from build123d import *

# Parameters (mm, degrees)
F0_R     = 8.382
F1_DEPTH = 12.7
F2_R     = 24.4449127013
F3_DEPTH = 25.4
F4_R     = 5.08
F6_DEPTH = 38.101


with BuildPart() as f1:
    # F0 (on Top) → F1 (new body)
    with BuildSketch(Plane.XY):
        with BuildLine():
            Line((10.7001249271, 26.4959987837), (0, 28.575))
            ThreePointArc((0, 28.575), (-28.575, 0), (0, -28.575))
            Line((0, -28.575), (10.7001249271, -26.4959987837))
            ThreePointArc((10.7001249271, -26.4959987837), (23.6884644373, -15.9808409542), (28.575, 0))
            ThreePointArc((28.575, 0), (23.6884644373, 15.9808409542), (10.7001249271, 26.4959987837))
        make_face()
        with BuildLine():
            ThreePointArc((10.7001249271, 26.4959987837), (5.4501128317, 28.0504348473), (0, 28.575))
            Line((0, 28.575), (10.7001249271, 26.4959987837))
        make_face()
        with BuildLine():
            Line((10.7001249271, -26.4959987837), (0, -28.575))
            ThreePointArc((0, -28.575), (5.4501128317, -28.0504348473), (10.7001249271, -26.4959987837))
        make_face()
        with BuildLine():
            Line((57.2391813175, 17.453603905), (10.7001249271, 26.4959987837))
            ThreePointArc((10.7001249271, 26.4959987837), (23.6884644373, 15.9808409542), (28.575, 0))
            ThreePointArc((28.575, 0), (23.6884644373, -15.9808409542), (10.7001249271, -26.4959987837))
            Line((10.7001249271, -26.4959987837), (57.2391813175, -17.453603905))
            ThreePointArc((57.2391813175, -17.453603905), (36.068, 0), (57.2391813175, 17.453603905))
        make_face()
        with BuildLine():
            ThreePointArc((71.628, 0), (67.5670306477, 11.3100220198), (57.2391813175, 17.453603905))
            ThreePointArc((57.2391813175, 17.453603905), (36.068, 0), (57.2391813175, -17.453603905))
            ThreePointArc((57.2391813175, -17.453603905), (67.5670306477, -11.3100220198), (71.628, 0))
        make_face()
        with Locations((53.848, 0)):
            Circle(F0_R, mode=Mode.SUBTRACT)
    extrude(amount=F1_DEPTH)

    # F2 (on face) → F3 (join)
    with BuildSketch(Plane.XY.offset(12.7)):
        Circle(F2_R)
    extrude(amount=F3_DEPTH)

    # F4
    f4_edges = [f1.edges().sort_by_distance(p)[0] for p in [
        (-24.444913, 0, 38.1),
    ]]
    fillet(f4_edges, radius=F4_R)

    # F5 (on face) → F6 (cut, through all)
    with BuildSketch(Plane.XY.offset(38.1)):
        with BuildLine():
            ThreePointArc((9.1075219166, -5.8424050607), (10.3833403237, -3.0441576954), (10.8203813405, 0))
            ThreePointArc((10.8203813405, 0), (10.5551078143, 2.3812499619), (9.7722941793, 4.6457420103))
            ThreePointArc((9.7722941793, 4.6457420103), (10.338343211, -0.6552772156), (9.1075219166, -5.8424050607))
        make_face()
        with BuildLine():
            ThreePointArc((9.7722941793, 4.6457420103), (10.5551078143, 2.3812499619), (10.8203813405, 0))
            ThreePointArc((10.8203813405, 0), (10.3833403237, -3.0441576954), (9.1075219166, -5.8424050607))
            Line((9.1075219166, -5.8424050607), (15.2793318605, -5.8424050607))
            Line((15.2793318605, -5.8424050607), (15.2793318605, 4.6457420103))
            Line((15.2793318605, 4.6457420103), (9.7722941793, 4.6457420103))
        make_face()
        with BuildLine():
            ThreePointArc((9.1075219166, -5.8424050607), (10.338343211, -0.6552772156), (9.7722941793, 4.6457420103))
            ThreePointArc((9.7722941793, 4.6457420103), (-10.7987115527, 0.6844568316), (9.1075219166, -5.8424050607))
        make_face()
    extrude(amount=-F6_DEPTH, mode=Mode.SUBTRACT)


solid = f1.part
For this review, take the finished solid that the model builds, in its own axes (mm). A direction names the side the tool comes from. Coordinates: 2 decimals unless noted, no trailing zeros. Order: outer loops, then holes, each group sorted by start corner. A loop starts at its lowest first (then second) coordinate and runs counter-clockwise, first axis right, second up. Notation, with made-up numbers: (17, 70.25) -> (25, 70.25) arc R15 ccw to (25, 88.25) -> close; hole circle Ø4 at (86, -31). An arc over 180 degrees is marked (long way). Return JSON: item names as keys, results as strings.
1. We need section A-A on z = 20. Write out the cut boundary in (x, y), and give its area (3 significant figures).
Answer block:
{"outline": "circle Ø48.89 at (0, 0); hole (9.11, -5.84) -> (15.28, -5.84) -> (15.28, 4.65) -> (9.77, 4.65) arc R10.82 ccw (long way) to start", "area": "1,460 mm²"}
2. For line 1 (X direction, y = -0.5, z = 8.5); line 2 (Y direction, x = 0, z = 28); line 3 (Z direction, x = 39, y = -8.5), list the stretches that pass through material, from the lowest coordinate up. Write a range as from..to.
Answer block:
{"line 1": "-28.57..-10.81, 15.28..45.48, 62.22..71.62", "line 2": "-24.44..-10.82, 10.82..24.44", "line 3": "0..12.7"}
3. The part is to be moulded in two halves that separate along X. For faces 1 (the flat face through (32, 0, 12.7)), 2 (the flat face through (13, 4.646, 19)), 3 (the cylindrical face through (-3.182, 24.237, 22.718)), 4 (the flat face through (12, -5.842, 19)), say which applies: +X half, -X half, draft (parallel to the pull), parting line (faces both ways), or undercut.
Answer block:
{"face 1": "draft", "face 2": "undercut", "face 3": "parting line", "face 4": "undercut"}
4. We need section C-C on x = 31. Write out the cut boundary in (y, z), and give its area (3 significant figures).
Answer block:
{"outline": "(-22.55, 0) -> (22.55, 0) -> (22.55, 12.7) -> (-22.55, 12.7) -> close", "area": "573 mm²"}
5. Machinability: for faces 5 (the flat face through (15.279, -1, 19)), 6 (the flat face through (21, 0, 0)), which of the approach directions +Z, -Z, +X, -X, +Y, -Y give a long, thin tool a straight path to every point of the face, cutting with its end or side? Answer none if there is none.
Answer block:
{"face 5": "+Z, -Z", "face 6": "-Z, +X, -X, +Y, -Y"}
6. We need section B-B on y = 6. State how many separate pieces and enclosed holes the cut face has, and give its area (3 significant figures).
Answer block:
{"separate pieces": "3", "enclosed holes": "0", "area": "1,610 mm²"}
7. For pin 1 Ø5 at (x, z) = (-7.5, 24) entering from +Y; pin 2 Ø10 at (x, z) = (31, 5) entering from -Y; pin 3 Ø5 at (x, z) = (11.5, 19) entering from +Y; pin 4 Ø13 at (x, y) = (0, 0) entering from -Z, all flat-tipped, find the tip position at first contact; note any pin that passes through.
Answer block:
{"pin 1": "y = 23.93", "pin 2": "y = -23.52", "pin 3": "y = 22.73", "pin 4": "through"}
